Source: three-view drawing plus pictorial views. Frame: mm from the lowest corner of the part. Coordinates: 2 decimals unless noted, no trailing zeros. Write each loop counter-clockwise with the first axis right and the second up, starting at its lowest first coordinate (ties: lowest second). Pieces come first, ordered by that corner, then holes. Notation, with made-up numbers: M 17.5,-22 L 58.5,-22 A25 ccw 58.5,1 Z; hole C 56,-27.75 d4. An arc over 180 degrees is marked long. Write item = value, one per line. Start each with the question number.
Item 1: Ray query, L1, parallel to X at y = 5.5, z = 3; L2, parallel to Y at x = 26, z = 15; L3, parallel to Z at x = 8, y = 11.5. Return the intervals inside material, ascending. Write a range as [from, to].
Item 2: Section C-C on x = 8. Output: boundary loops of the cut face in (y, z).
Item 3: Section B-B on z = 27. Output: boundary loops of the cut face in (x, y).
Item 4: Section D-D on y = 16.5. Output: boundary loops of the cut face in (x, z), plus the area to 3 significant figures.
Item 5: Pull-direction query (Y, two-part tool) for the marked faces 1, 2 and 3; classes: +Y half, -Y half, draft (parallel to the pull), parting line (faces both ways), or undercut.
Item 6: Section A-A on y = 11. Output: boundary loops of the cut face in (x, z), plus the area to 3 significant figures.
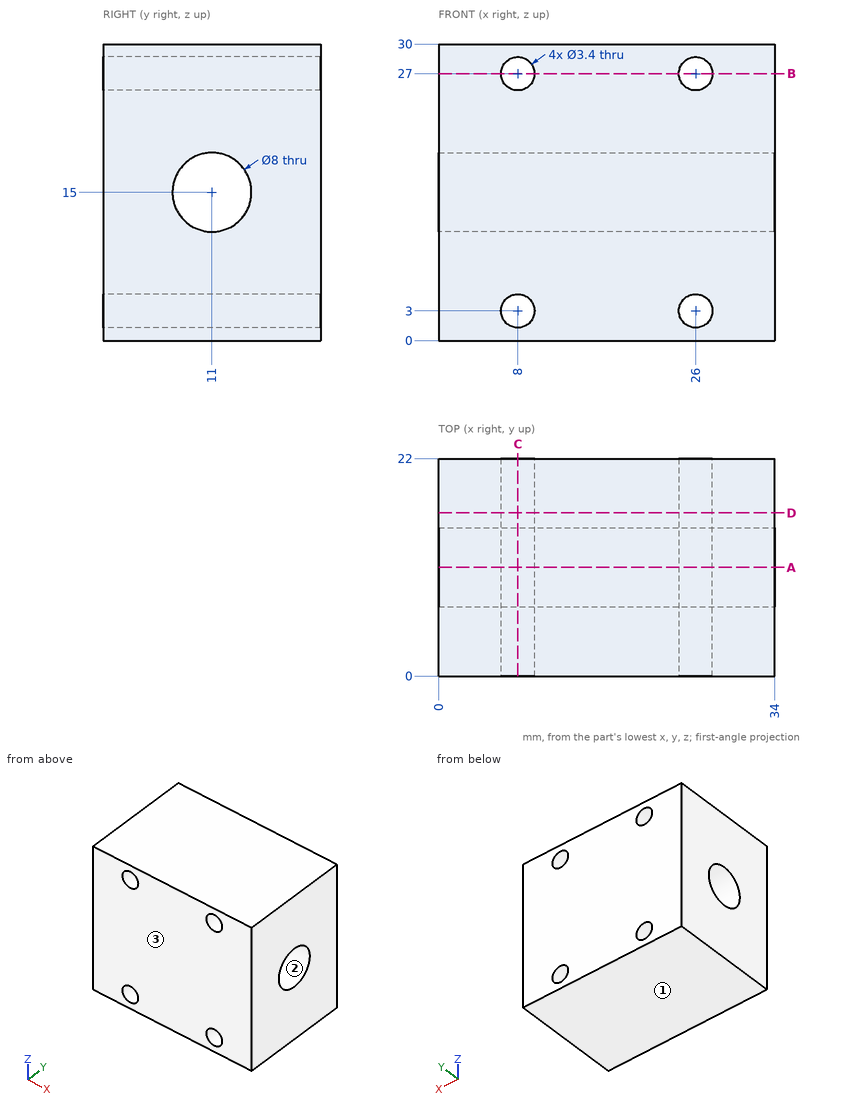
Responses:
q1.L1 = [0, 6.3], [9.7, 24.3], [27.7, 34]
q1.L2 = [0, 7], [15, 22]
q1.L3 = [0, 1.3], [4.7, 11.03], [18.97, 25.3], [28.7, 30]
q2.outline = M 0,0 L 22,0 L 22,1.3 L 0,1.3 Z; M 0,4.7 L 22,4.7 L 22,25.3 L 0,25.3 Z; M 0,28.7 L 22,28.7 L 22,30 L 0,30 Z; hole C 11,15 d8
q3.outline = M 0,0 L 6.3,0 L 6.3,22 L 0,22 Z; M 9.7,0 L 24.3,0 L 24.3,22 L 9.7,22 Z; M 27.7,0 L 34,0 L 34,22 L 27.7,22 Z
q4.outline = M 0,0 L 34,0 L 34,30 L 0,30 Z; hole C 8,3 d3.4; hole C 8,27 d3.4; hole C 26,3 d3.4; hole C 26,27 d3.4
q4.area = 984 mm²
q5.face_1 = draft
q5.face_2 = undercut
q5.face_3 = -Y half
q6.outline = M 0,0 L 34,0 L 34,11 L 0,11 Z; M 0,19 L 34,19 L 34,30 L 0,30 Z; hole C 8,3 d3.4; hole C 8,27 d3.4; hole C 26,3 d3.4; hole C 26,27 d3.4
q6.area = 712 mm²
